from build123d import *
from OCP.BRepFilletAPI import BRepFilletAPI_MakeChamfer

# Parameters (mm, degrees)
SKETCH1_W           = 15
SKETCH1_H           = 20
SKETCH1_R           = 1.7
BOSS_EXTRUDE1_DEPTH = 8
SKETCH2_R           = 3.5
CUT_EXTRUDE1_DEPTH  = 5
CUT_EXTRUDE2_DEPTH  = 20.723082923
CHAMFER1_SIZE       = 1
CHAMFER1_SIZE2      = 0.849836586
CHAMFER1_SIZE2_2    = 1.274754878


with BuildPart() as part:
    # Sketch1 → Boss-Extrude1 (new body)
    with BuildSketch(Plane.XY):
        Rectangle(SKETCH1_W, SKETCH1_H)
        Circle(SKETCH1_R, mode=Mode.SUBTRACT)
    extrude(amount=BOSS_EXTRUDE1_DEPTH)

    # Sketch2 → Cut-Extrude1 (cut)
    with BuildSketch(Plane.XY.offset(8)):
        Circle(SKETCH2_R)
    extrude(amount=-CUT_EXTRUDE1_DEPTH, mode=Mode.SUBTRACT)

    # Sketch3 → Cut-Extrude2 (cut, through all)
    with BuildSketch(Plane(origin=(7.5, 0, 0), x_dir=(0, 0, -1), z_dir=(1, 0, 0))):
        Polygon((-8, 10), (-4, -10), (-8, -10), align=None)
    extrude(amount=-CUT_EXTRUDE2_DEPTH, mode=Mode.SUBTRACT)

    # Chamfer1: one chamfer whose edges measure the first distance from different faces: ONE call of the kernel's chamfer builder (chamfer() names one face for all edges)
    chamfer1_edges_1 = [part.edges().sort_by_distance(p)[0] for p in [
        (0, 10, 8),
    ]]
    chamfer1_side_1 = [part.faces().sort_by_distance(p)[0] for p in [
        (0, 10, 4),
    ]]
    chamfer1_edges_2 = [part.edges().sort_by_distance(p)[0] for p in [
        (-7.5, 0, 6),
        (7.5, 0, 6),
    ]]
    chamfer1_edges_3 = [part.edges().sort_by_distance(p)[0] for p in [
        (0, -10, 4),
    ]]
    chamfer1_side_3 = [part.faces().sort_by_distance(p)[0] for p in [
        (0, -10, 2),
    ]]
    chamfer1 = BRepFilletAPI_MakeChamfer(part.part.solid().wrapped)
    for e in chamfer1_edges_1:
        chamfer1.Add(CHAMFER1_SIZE, CHAMFER1_SIZE2, e.wrapped, chamfer1_side_1[0].wrapped)  # the first distance lies on this face
    for e in chamfer1_edges_2:
        chamfer1.Add(CHAMFER1_SIZE, e.wrapped)
    for e in chamfer1_edges_3:
        chamfer1.Add(CHAMFER1_SIZE, CHAMFER1_SIZE2_2, e.wrapped, chamfer1_side_3[0].wrapped)  # the first distance lies on this face
    add(Compound.cast(chamfer1.Shape()), mode=Mode.REPLACE)


solid = part.part
CAD build for the part. Positions are in the model's coordinates, mm. A direction names the side the tool comes from. Coordinates: 2 decimals unless noted, no trailing zeros. Write each loop counter-clockwise with the first axis right and the second up, starting at its lowest first coordinate (ties: lowest second). Pieces come first, ordered by that corner, then holes. Notation, with made-up numbers: M 12.25,-13.75 L 57.25,-13.75 A25 cw 57.25,4.25 Z; hole C -28.5,25.25 d3. An arc over 180 degrees is marked long. Return JSON: item names as keys, results as strings.
Item 1: Slice it at A-A, the plane x = 0. Write the cut outline in (y, z).
Findings below:
{"outline": "M -10,0 L -1.7,0 L -1.7,3 L -3.5,3 L -3.5,5.3 L -8.75,4.25 L -10,3 Z; M 1.7,0 L 10,0 L 10,7 L 9.17,7.83 L 3.5,6.7 L 3.5,3 L 1.7,3 Z"}
Item 2: Drop flat-ended pins along their axis: pin 1 Ø2 at (x, y) = (0, 8) entering from +Z; pin 2 Ø5.5 at (x, y) = (0, 1) entering from +Z; pin 3 Ø1.5 at (x, y) = (-4, -4) entering from +Z. Give the stop position or say it passes through.
Findings below:
{"pin 1": "stops at z = 7.8", "pin 2": "stops at z = 6.75", "pin 3": "stops at z = 5.35"}
Item 3: Slice it at B-B, the plane y = 0. Write the cut outline in (x, z), and give its area (3 significant figures).
Findings below:
{"outline": "M -7.5,0 L -1.7,0 L -1.7,3 L -3.5,3 L -3.5,6 L -6.5,6 L -7.5,4.98 Z; M 1.7,0 L 7.5,0 L 7.5,4.98 L 6.5,6 L 3.5,6 L 3.5,3 L 1.7,3 Z", "area": "57.8 mm2"}
Item 4: Slice it at D-D, the plane x = 6. Write the cut outline in (y, z), and give its area (3 significant figures).
Findings below:
{"outline": "M -10,0 L 10,0 L 10,7 L 9.17,7.83 L -8.75,4.25 L -10,3 Z", "area": "119 mm2"}
Item 5: Slice it at C-C, the plane z = 3.75. Write the cut outline in (x, y).
Findings below:
{"outline": "M -7.5,-6.15 L -6.89,-9.25 L 6.89,-9.25 L 7.5,-6.15 L 7.5,10 L -7.5,10 Z; hole C 0,0 d7"}
Item 6: Which spindle directions (+Z, -Z, +X, -X, +Y, -Y) get a long thin tool onto all of the face, cutting with end or side? Do faces 4 (the cylindrical face through (1.88, 2.95, 4.46)), 5 (the flat face through (0, 10, 3)). Say none if no direction does.
Findings below:
{"face 4": "+Z", "face 5": "+Z, -Z, +X, -X, +Y"}
Item 7: Two-plate mould, pull along Y, no slides. Class faces 1 (the flat face through (-2, 0, 0)), 2 (the flat face through (0, -10, 1)), 3 (the cylindrical face through (-0.37, -1.66, 1.48)): +Y half, -Y half, draft (parallel to the pull), parting line (faces both ways), or undercut.
Findings below:
{"face 1": "draft", "face 2": "-Y half", "face 3": "undercut"}
Item 8: Probe line 1 (X direction, y = 0, z = 2.25); line 2 (Y direction, x = 0, z = 1.25); line 3 (X direction, y = 0, z = 4.65). List the from-to ranges inside material, lowest first. Write a range as from..to.
Findings below:
{"line 1": "x = -7.5..-1.7, 1.7..7.5", "line 2": "y = -10..-1.7, 1.7..10", "line 3": "x = -7.5..-3.5, 3.5..7.5"}
